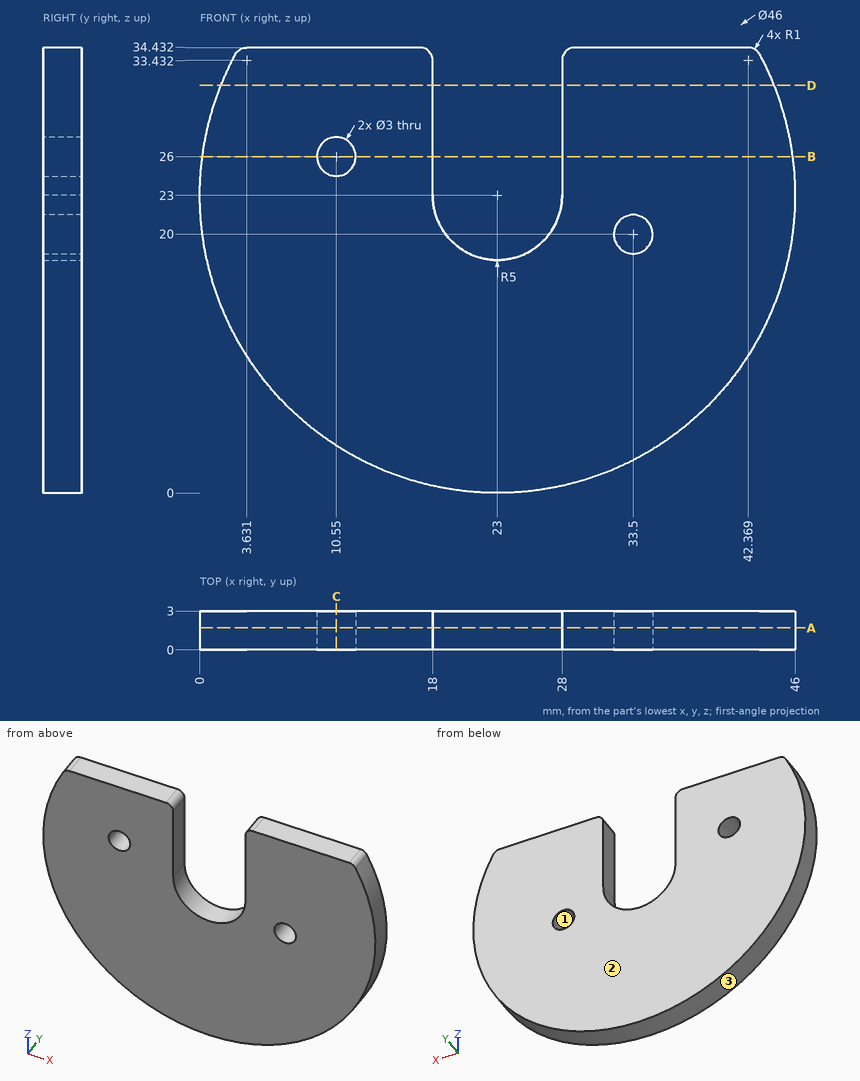
Drawing for the job (mm, zero at the part's lowest x, y, z). Give positions to 0.01 mm unless a question says otherwise; leave off trailing zeros. Loops run counter-clockwise (first coordinate to the right, second up) from the corner with the lowest first, then second, coordinate; pieces in that order, holes last.
Item 1: Slice it at D-D (z = 31.5). Write the cut outline in (x, y).
Check values:
outline: (1.63, 0) - (18, 0) - (18, 3) - (1.63, 3) - close; (28, 0) - (44.37, 0) - (44.37, 3) - (28, 3) - close
Item 2: Drop a flat-ended pin along its axis: P1, Ø0.9, axis at y = 1, z = 28.5, coming from the +X side. Give the stop position or say it passes through.
Check values:
P1: stops at x = 45.44
Item 3: Mould opens along X. For the marked faces 1, 2 and 3 say: +X half, -X half, draft (parallel to the pull), parting line (faces both ways), or undercut.
Check values:
face 1: undercut
face 2: draft
face 3: parting line
Item 4: Drill centre lines: line 1 along X through (y, z) = (2.05, 20) (1 decimal); line 2 along X through (y, z) = (1.25, 26.5) (1 decimal); line 3 along X through (y, z) = (2, 24). Where is each one in solid material? Low to high.
Check values:
line 1: x = 0.2 to 19, 27 to 32, 35 to 45.8
line 2: x = 0.3 to 9.1, 12 to 18, 28 to 45.7
line 3: x = 0.02 to 18, 28 to 45.98
Item 5: Slice it at A-A (y = 1.7). Write the cut outline in (x, z), plus the area to 3 significant figures.
Check values:
outline: (2.75, 33.91) arc R23 ccw (long way) to (43.25, 33.91) arc R1 ccw to (42.37, 34.43) - (29, 34.43) arc R1 ccw to (28, 33.43) - (28, 23.07) arc R5 cw (long way) to (18, 23.07) - (18, 33.43) arc R1 ccw to (17, 34.43) - (3.63, 34.43) arc R1 ccw to start; hole circle Ø3 at (10.55, 26); hole circle Ø3 at (33.5, 20)
area: 1,170 mm2
Item 6: Slice it at C-C (x = 10.55). Write the cut outline in (y, z).
Check values:
outline: (0, 3.66) - (3, 3.66) - (3, 24.5) - (0, 24.5) - close; (0, 27.5) - (3, 27.5) - (3, 34.43) - (0, 34.43) - close
Item 7: Slice it at B-B (z = 26). Write the cut outline in (x, y).
Check values:
outline: (0.2, 0) - (9.05, 0) - (9.05, 3) - (0.2, 3) - close; (12.05, 0) - (18, 0) - (18, 3) - (12.05, 3) - close; (28, 0) - (45.8, 0) - (45.8, 3) - (28, 3) - close
